For this review, take the finished solid that the model builds, in its own axes (mm). A direction names the side the tool comes from. Round coordinates to 2 decimals unless told otherwise and drop trailing zeros. Order: outer loops, then holes, each group sorted by start corner. A loop starts at its lowest first (then second) coordinate and runs counter-clockwise, first axis right, second up. Notation, with made-up numbers: M 89,52 L 121,52 A22 ccw 121,60 Z; hole C -31.75,60 d5. An arc over 180 degrees is marked long. Use a Markdown table: item, result.
from build123d import *

# Parameters (mm, degrees)
F0_R     = 15
F1_DEPTH = 22.5
F2_DEPTH = 8.5
F3_DEPTH = 31
F5_R     = 15
F6_DEPTH = 18


# Not quite as in the source:
# - a pattern or mirror of a feature is missing from the dataset's text; its kind, count and spacing are read off the source's solid


with BuildPart() as f1:
    # F0 (on Front) → F1 (new body, symmetric)
    with BuildSketch(Plane.XZ):
        with BuildLine():
            ThreePointArc((0, -25), (17.6776695297, -17.6776695297), (25, 0))
            ThreePointArc((25, 0), (17.6776695297, 17.6776695297), (0, 25))
            ThreePointArc((0, 25), (-25, 0), (0, -25))
        make_face()
        Circle(F0_R, mode=Mode.SUBTRACT)
    extrude(amount=F1_DEPTH, both=True)

    # F0 (on Front) → F2 (join, symmetric)
    with BuildSketch(Plane.XZ):
        with BuildLine():
            ThreePointArc((0, 25), (17.6776695297, 17.6776695297), (25, 0))
            ThreePointArc((25, 0), (17.6776695297, -17.6776695297), (0, -25))
            Line((0, -25), (70, -25))
            Line((70, -25), (70, 25))
            Line((70, 25), (0, 25))
        make_face()
    extrude(amount=F2_DEPTH, both=True)

    # F0 (on Front) → F3 (join, symmetric)
    with BuildSketch(Plane.XZ):
        Polygon((80, 25), (70, 25), (70, -25), (80, -25), (80, 0), align=None)
    extrude(amount=F3_DEPTH, both=True)

    # F5 (on offset) → F6 (join)
    with BuildSketch(Plane.XZ.offset(35)):
        with BuildLine():
            ThreePointArc((93.4168760482, -25), (124.1863716546, -26.4338203685), (140, 0))
            ThreePointArc((140, 0), (124.1863716546, 26.4338203685), (93.4168760482, 25))
            ThreePointArc((93.4168760482, 25), (83.5661796315, 14.1863716546), (80, 0))
            ThreePointArc((80, 0), (83.5661796315, -14.1863716546), (93.4168760482, -25))
        make_face()
        with Locations((110, 0)):
            Circle(F5_R, mode=Mode.SUBTRACT)
        with BuildLine():
            ThreePointArc((80, 0), (83.5661796315, 14.1863716546), (93.4168760482, 25))
            Line((93.4168760482, 25), (80, 25))
            Line((80, 25), (80, 0))
        make_face()
        with BuildLine():
            Line((80, -25), (93.4168760482, -25))
            ThreePointArc((93.4168760482, -25), (83.5661796315, -14.1863716546), (80, 0))
            Line((80, 0), (80, -25))
        make_face()
    f6 = extrude(amount=-F6_DEPTH)

    # F6_copies: F6 across plane
    add(f6.mirror(Plane.ZX))


solid = f1.part
Q1. Add section D-D (y = -29). Write out the cut boundary in (x, z), then the cut area to 3 significant figures.
Determined:
| item | result |
|---|---|
| outline | M 70,-25 L 93.42,-25 A30 ccw long 93.42,25 L 70,25 Z; hole C 110,0 d30 |
| area | 2,820 mm^2 |
Q2. Add section A-A (x = 110). Write out the cut boundary in (y, z), then the cut area to 3 significant figures.
Determined:
| item | result |
|---|---|
| outline | M -35,-30 L -17,-30 L -17,-15 L -35,-15 Z; M -35,15 L -17,15 L -17,30 L -35,30 Z; M 17,-30 L 35,-30 L 35,-15 L 17,-15 Z; M 17,15 L 35,15 L 35,30 L 17,30 Z |
| area | 1,080 mm^2 |
Q3. Wall thickness on line 1 along Z through (x, y) = (0, -6); line 2 along Y through (x, z) = (89.5, 17.5); line 3 along Z through (x, y) = (110, 24): over which ranges is each line inside the solid? List them lowest first. Write a range as [from, to].
Determined:
| item | result |
|---|---|
| line 1 | z = [-25, -15], [15, 25] |
| line 2 | y = [-35, -17], [17, 35] |
| line 3 | z = [-30, -15], [15, 30] |
Q4. Add section B-B (y = 14). Write out the cut boundary in (x, z).
Determined:
| item | result |
|---|---|
| outline | C 0,0 d50; M 70,-25 L 80,-25 L 80,25 L 70,25 Z; hole C 0,0 d30 |
Q5. Add section C-C (z = -3.5). Give the number of separate pieces and of enclosed holes in the cut face, then the cut area to 3 significant figures.
Determined:
| item | result |
|---|---|
| separate pieces | 4 |
| enclosed holes | 0 |
| area | 3,410 mm^2 |
Q6. Draft analysis for pull direction X (two halves, no side actions). For faces 1 (the flat face through (96, 35, -6)), 2 (the flat face through (70, 20, 0)), 3 (the flat face through (80, -33, 0)), state which applies: pulls with the +X half, pulls with the -X half, needs draft (parallel to the pull), parting line crosses it, or undercut.
Determined:
| item | result |
|---|---|
| face 1 | needs draft |
| face 2 | undercut |
| face 3 | pulls with the -X half |
Q7. Clearance check with flat-ended pins moving along their axes: pin 1 (1 mm diameter, centred on y = 4.5, z = -15, fed in from +X); pin 2 (10 mm diameter, centred on y = -18, z = 7.5, fed in from +X); pin 3 (8 mm diameter, centred on x = -7, y = 1.5, fed in from -Z); pin 4 (18 mm diameter, centred on x = 106.5, z = -7, fed in from +Y). State where each tip first meets the part, or that it passes through.
Determined:
| item | result |
|---|---|
| pin 1 | stops at x = 80 |
| pin 2 | stops at x = 139.9 |
| pin 3 | stops at z = -24.82 |
| pin 4 | stops at y = 35 |
Q8. Machinability: for faces 4 (the flat face through (70, -20, 0)), 5 (the flat face through (80, 0, 0)), 6 (the flat face through (75, -31, 0)), which of the approach directions +Z, -Z, +X, -X, +Y, -Y give a long, thin tool a straight path to every point of the face, cutting with its end or side? Answer none if there is none.
Determined:
| item | result |
|---|---|
| face 4 | +Z, -Z, -Y |
| face 5 | +Z, -Z, +X |
| face 6 | +Z, -Z, -X, -Y |
